```python
from build123d import *

# Parameters (mm, degrees)
SALIENTE_EXTRUIR1_DEPTH = 3
CROQUIS2_R              = 6
CORTAR_EXTRUIR1_DEPTH   = 3


with BuildPart() as part:
    # Croquis1 → Saliente-Extruir1 (new body)
    with BuildSketch(Plane.XY):
        with BuildLine():
            Line((-48.541019662, 35.267115138), (-60.676274578, 44.083893922))
            ThreePointArc((-60.676274578, 44.083893922), (-33.17983972, 62.875244761), (0, 60))
            ThreePointArc((0, 60), (59.261300436, -9.386067902), (-18.541019662, -57.063390978))
            Line((-18.541019662, -57.063390978), (-23.176274578, -71.329238722))
            ThreePointArc((-23.176274578, -71.329238722), (-49.544776899, -50.985421932), (-57.063390978, -18.541019662))
            ThreePointArc((-57.063390978, -18.541019662), (-59.261300436, 9.386067902), (-48.541019662, 35.267115138))
        make_face()
    extrude(amount=SALIENTE_EXTRUIR1_DEPTH)

    # Croquis2 → Cortar-Extruir1 (cut)
    with BuildSketch(Plane.XY.offset(3)):
        Circle(CROQUIS2_R)
    extrude(amount=-CORTAR_EXTRUIR1_DEPTH, mode=Mode.SUBTRACT)


solid = part.part
```
Model file for the job. Use its own axes, mm. A direction names the side the tool comes from. Coordinates: 2 decimals unless noted, no trailing zeros. Loops run counter-clockwise (first coordinate to the right, second up) from the corner with the lowest first, then second, coordinate; pieces in that order, holes last. Notation, with made-up numbers: (59.25, 84.5) -> (88.25, 84.5) arc R26 ccw to (88.25, 121.5) -> close; hole circle Ø7 at (57.25, 0.5). An arc over 180 degrees is marked (long way). Answer as a JSON object with one key per item and string values.
Q1. Pull direction Y, two halves, no side cores. Call faces 1 (the cylindrical face through (59.47, -7.95, 1.48)), 2 (the flat face through (-13, -2, 0)), 3 (the cylindrical face through (-59.322, 8.995, 1.479)), 4 (the flat face through (-20.826, -64.096, 1.479)): released by +Y, released by -Y, zero draft, split by the parting line, or undercut.
Report:
{"face 1": "split by the parting line", "face 2": "zero draft", "face 3": "undercut", "face 4": "released by -Y"}
Q2. Probe probe 1 along Y at (x, z) = (-4, 1.7); probe 2 along Y at (x, z) = (-3.5, 0.9); probe 3 along Y at (x, z) = (18, 1.6). List the from-to ranges inside material, lowest first.
Report:
{"probe 1": "y = -59.87 to -4.47, 4.47 to 61.62", "probe 2": "y = -59.9 to -4.87, 4.87 to 61.44", "probe 3": "y = -57.24 to 57.24"}
Q3. Flat gauge pin, fed straight in: P1, Ø1, axis at y = 24.5, z = 2.5, coming from the +X side. Where does the tip first touch, or does it go through?
Report:
{"P1": "stops at x = 54.99"}
Q4. Cut at A-A (z = 0.5). List the corners of the cut face in (x, y).
Report:
{"outline": "(-60.68, 44.08) -> (-48.54, 35.27) arc R60 ccw to (-57.06, -18.54) arc R49.52 ccw to (-23.18, -71.33) -> (-18.54, -57.06) arc R60 ccw (long way) to (0, 60) arc R49.52 ccw to start; hole circle Ø12 at (0, 0)"}
Q5. Cut at B-B (y = 0). List the corners of the cut face in (x, z).
Report:
{"outline": "(-60, 0) -> (-6, 0) -> (-6, 3) -> (-60, 3) -> close; (6, 0) -> (60, 0) -> (60, 3) -> (6, 3) -> close"}
Q6. Cut at D-D (y = -28.5). List the corners of the cut face in (x, z).
Report:
{"outline": "(-57.21, 0) -> (52.8, 0) -> (52.8, 3) -> (-57.21, 3) -> close"}
Q7. Cut at C-C (x = 39). List the corners of the cut face in (y, z), and give its area (3 significant figures).
Report:
{"outline": "(-45.6, 0) -> (45.6, 0) -> (45.6, 3) -> (-45.6, 3) -> close", "area": "274 mm2"}
Q8. 3-axis set-ups, long thin cutter, end or side, ignore diameter. For faces 5 (the flat face through (-54.52, 39.61, 1.48)), 6 (the flat face through (-13, -2, 3)): which of +Z, -Z, +X, -X, +Y, -Y reach the whole face in a straight line?
Report:
{"face 5": "+Z, -Z, -X", "face 6": "+Z, +X, -X, +Y, -Y"}
